from build123d import *

# Parameters (mm, degrees)
CUT_EXTRUDE1_START = -61
CUT_EXTRUDE1_DEPTH = 61


# Read off the part's stored shape, not the designer's step: Cut-Extrude1
with BuildPart() as part:
    # Sketch1 → Loft1 section 0
    with BuildSketch(Plane(origin=(0, 0, 0), x_dir=(1, 0, 0), z_dir=(0, 1, 0))):
        with BuildLine():
            Line((0, 0), (58.2, 0))
            Line((58.2, 0), (58.2, 61))
            Line((58.2, 61), (0, 61))
            Line((0, 61), (0, 0))
        make_face()
    # Sketch2 → Loft1 section 1
    with BuildSketch(Plane(origin=(0, 6.099999992, 0), x_dir=(1, 0, 0), z_dir=(0, 1, 0))):
        with BuildLine():
            Line((-4.8, 61), (63, 61))
            Line((63, 61), (63, 0))
            Line((63, 0), (-4.8, 0))
            Line((-4.8, 0), (-4.8, 61))
        make_face()
    loft()

    # Cut-Extrude1 outline → Cut-Extrude1 (cut)
    with BuildSketch(Plane.XY.offset(CUT_EXTRUDE1_START)):
        Polygon((60.861632844, 6.099999992), (56.132109475, 6.099999992), (54.298183465, 0.936182189), (57.189353849, 0.936182189), align=None)
        Polygon((54.750384399, 6.099999992), (52.107282262, 6.099999992), (50.541618156, 0.936182189), (52.916458389, 0.936182189), align=None)
        Polygon((51.025910518, 6.099999992), (47.612762768, 6.099999992), (46.735990868, 0.936182189), (49.460246412, 0.936182189), align=None)
        Polygon((46.328918201, 6.099999992), (43.729915785, 6.099999992), (42.853143886, 0.936182189), (45.452146301, 0.936182189), align=None)
        Polygon((14.470084215, 6.099999992), (11.871081799, 6.099999992), (12.747853699, 0.936182189), (15.346856114, 0.936182189), align=None)
        Polygon((10.587237232, 6.099999992), (7.174089482, 6.099999992), (8.739753588, 0.936182189), (11.464009132, 0.936182189), align=None)
        Polygon((6.092717738, 6.099999992), (3.449615601, 6.099999992), (5.283541611, 0.936182189), (7.658381844, 0.936182189), align=None)
        Polygon((1.010646151, 0.936182189), (3.901816535, 0.936182189), (2.067890525, 6.099999992), (-2.661632844, 6.099999992), align=None)
    extrude(amount=CUT_EXTRUDE1_DEPTH, mode=Mode.SUBTRACT)


solid = part.part
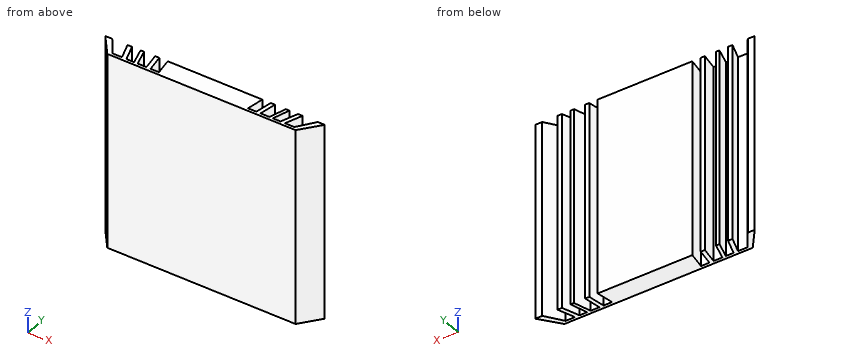
Source: CAD feature listing. Evaluate the final solid. Frame: model axes, mm. Coordinates: 2 decimals unless noted, no trailing zeros. One line per question, with ' | ' between items.
1) Line query: line 1 along Y through (x, z) = (9.5, -56); line 2 along X through (y, z) = (0.5, -57.5); line 3 along X through (y, z) = (0.75, -11.5). Output: solid intervals per line, ascending.
Report:
line 1: y = 0 to 0.94 | line 2: x = -0.39 to 58.59 | line 3: x = -0.59 to 58.79
2) First-contact query: P1, Ø0.8, axis at x = 13.5, z = -20.5, coming from the +Y side; P2, Ø3, axis at y = 1, z = -46.5, coming from the +X side; P3, Ø1, axis at y = 4.5, z = -24.5, coming from the -X side. Flat tips, straight axial feed; report the tip coordinate or a pass-through.
Report:
P1: stops at y = 0.94 | P2: stops at x = 60.17 | P3: stops at x = -3.93
3) Section A-A, the plane y = 2. Give the number of separate pieces and of enclosed holes in the cut face, then the cut area to 3 significant figures.
Report:
separate pieces: 9 | enclosed holes: 0 | area: 2,380 mm²
